Input: part model. Units: mm. Frame: model coordinates. Face numbers are marked on the shaded views. A direction names the side the tool comes from. Coordinates: 2 decimals unless noted, no trailing zeros. Write each loop counter-clockwise with the first axis right and the second up, starting at its lowest first coordinate (ties: lowest second). Pieces come first, ordered by that corner, then holes.
from build123d import *

# Parameters (mm, degrees)
SKETCH_1_W          = 107.18
SKETCH_1_H          = 107.18
EXTRUDE_1_DEPTH     = 27
SKETCH_2_W          = 92
SKETCH_2_H          = 92
CUT_EXTRUDE_1_DEPTH = 23
SKETCH_3_R          = 6
CUT_EXTRUDE_2_DEPTH = 123.835013331
EXTRUDE_3_DEPTH     = 6
SKETCH_7_R          = 2
EXTRUDE_4_DEPTH     = 3


with BuildPart() as part:
    # 草图1 → 凸台-拉伸1 (new body)
    with BuildSketch(Plane.XY):
        Rectangle(SKETCH_1_W, SKETCH_1_H)
    extrude(amount=EXTRUDE_1_DEPTH)

    # 草图2 → 切除-拉伸1 (cut)
    with BuildSketch(Plane.XY.offset(27)):
        Rectangle(SKETCH_2_W, SKETCH_2_H)
    extrude(amount=-CUT_EXTRUDE_1_DEPTH, mode=Mode.SUBTRACT)

    # 草图3 → 切除-拉伸2 (cut, through all)
    with BuildSketch(Plane(origin=(0, 53.59, 0), x_dir=(1, 0, 0), z_dir=(0, 1, 0))):
        with Locations((0, -27)):
            Circle(SKETCH_3_R)
    extrude(amount=-CUT_EXTRUDE_2_DEPTH, mode=Mode.SUBTRACT)

    # 草图5 → 凸台-拉伸3 (add)
    with BuildSketch(Plane(origin=(53.59, 0, 0), x_dir=(0, 0, -1), z_dir=(1, 0, 0))):
        with BuildLine():
            ThreePointArc((-27, -15), (-12, 0), (-27, 15))
            Line((-27, 15), (-27, 12.5))
            ThreePointArc((-27, 12.5), (-14.5, 0), (-27, -12.5))
            Line((-27, -12.5), (-27, -15))
        make_face()
    extrude(amount=EXTRUDE_3_DEPTH)

    # 草图7 → 凸台-拉伸4 (add)
    # profile 1 of 4: a face of its own
    with BuildSketch(Plane.XY.offset(27)):
        with BuildLine():
            Line((-56.5, 53.59), (-49.473493433, 53.59))
            Line((-49.473493433, 53.59), (-49.473493433, 47.59))
            Line((-49.473493433, 47.59), (-56.5, 47.59))
            ThreePointArc((-56.5, 47.59), (-59.5, 50.59), (-56.5, 53.59))
        make_face()
        with Locations((-56.5, 50.59)):
            Circle(SKETCH_7_R, mode=Mode.SUBTRACT)
    # profile 2 of 4: a face of its own
    with BuildSketch(Plane.XY.offset(27)):
        with BuildLine():
            Line((51.172302286, 53.59), (56.5, 53.59))
            ThreePointArc((56.5, 53.59), (59.5, 50.59), (56.5, 47.59))
            Line((56.5, 47.59), (51.172302286, 47.59))
            Line((51.172302286, 47.59), (51.172302286, 53.59))
        make_face()
        with Locations((56.5, 50.59)):
            Circle(SKETCH_7_R, mode=Mode.SUBTRACT)
    # profile 3 of 4: a face of its own
    with BuildSketch(Plane.XY.offset(27)):
        with BuildLine():
            Line((51.172302286, -47.59), (56.5, -47.59))
            ThreePointArc((56.5, -47.59), (59.5, -50.59), (56.5, -53.59))
            Line((56.5, -53.59), (51.172302286, -53.59))
            Line((51.172302286, -53.59), (51.172302286, -47.59))
        make_face()
        with Locations(Location((56.5, -50.59, 0), (0, 0, 180))):
            Circle(SKETCH_7_R, mode=Mode.SUBTRACT)
    # profile 4 of 4: a face of its own
    with BuildSketch(Plane.XY.offset(27)):
        with BuildLine():
            Line((-49.473493433, -53.59), (-49.473493433, -47.59))
            Line((-49.473493433, -47.59), (-56.5, -47.59))
            ThreePointArc((-56.5, -47.59), (-59.5, -50.59), (-56.5, -53.59))
            Line((-56.5, -53.59), (-49.473493433, -53.59))
        make_face()
        with Locations(Location((-56.5, -50.59, 0), (0, 0, 180))):
            Circle(SKETCH_7_R, mode=Mode.SUBTRACT)
    extrude(amount=-EXTRUDE_4_DEPTH)


solid = part.part
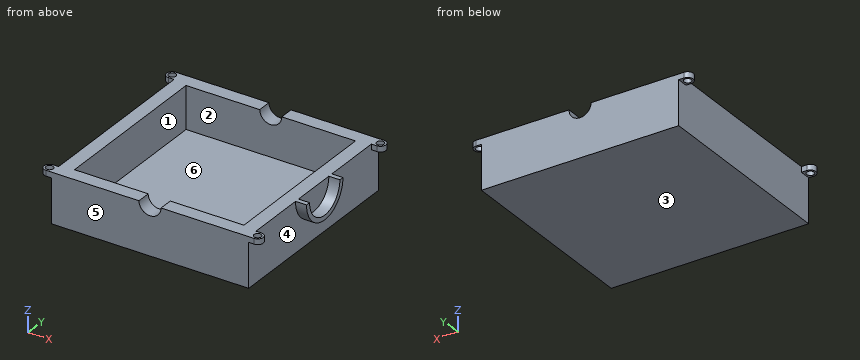
Item 1: Section query C-C, the plane y = 0. Return loops of the section in (x, z).
Item 2: Section query B-B, the plane z = 6.75. Return loops of the section in (x, y).
Item 3: Pin query (flat end, axial travel): pin 1 Ø1.8 at (x, y) = (-57.5, -51.5) entering from -Z; pin 2 Ø5 at (y, z) = (-38.5, 15.5) entering from -X; pin 3 Ø3 at (x, y) = (-56.5, 50.59) entering from -Z (3 decimals); pin 4 Ø2 at (y, z) = (40, 5) entering from +X. Return the tip coordinate at first contact, or that it passes through.
Item 4: Pull-direction query (X, two-part tool) for the marked faces 1, 2, 3 and 4; classes: released by +X, released by -X, zero draft, split by the parting line, or undercut.
Item 5: Access query for the marked faces 5 and 6. Directions: +Z, -Z, +X, -X, +Y, -Y. A direction counts if a zero-diameter tool reaches every point of the face in a straight line with its end or side. Return the directions, or none.
Item 6: Section query A-A, the plane y = 50.59. Return loops of the section in (x, z), then the cut area to 3 significant figures.
Item 7: Material intervals for line 1 (Y direction, x = -56.5, z = 26.3); line 2 (Y direction, x = -19, z = 21.5), sorted ascending.
Item 8: Section query D-D, the plane x = 0. Return loops of the section in (y, z).
The answers:
1. outline: (-53.59, 0) - (53.59, 0) - (53.59, 12) - (59.59, 12) - (59.59, 14.5) - (53.59, 14.5) - (53.59, 27) - (46, 27) - (46, 4) - (-46, 4) - (-46, 27) - (-53.59, 27) - close
2. outline: (-53.59, -53.59) - (53.59, -53.59) - (53.59, 53.59) - (-53.59, 53.59) - close; hole (-46, -46) - (46, -46) - (46, 46) - (-46, 46) - close
3. pin 1: stops at z = 24
3. pin 2: stops at x = -53.59
3. pin 3: passes through
3. pin 4: stops at x = 53.59
4. face 1: undercut
4. face 2: undercut
4. face 3: zero draft
4. face 4: released by +X
5. face 5: +Z, -Z, +X, -X, -Y
5. face 6: +Z
6. outline: (-59.5, 24) - (-58.5, 24) - (-58.5, 27) - (-59.5, 27) - close; (-54.5, 24) - (-53.59, 24) - (-53.59, 0) - (53.59, 0) - (53.59, 24) - (54.5, 24) - (54.5, 27) - (6, 27) arc R6 cw to (-6, 27) - (-54.5, 27) - close; (58.5, 24) - (59.5, 24) - (59.5, 27) - (58.5, 27) - close
6. area: 2,850 mm2
7. line 1: y = -53.59 to -52.59, -48.59 to -47.59, 47.59 to 48.59, 52.59 to 53.59
7. line 2: y = -53.59 to -46, 46 to 53.59
8. outline: (-53.59, 0) - (53.59, 0) - (53.59, 21) - (46, 21) - (46, 4) - (-46, 4) - (-46, 21) - (-53.59, 21) - close
